Part model, mm, in its own coordinate system. Coordinates: 2 decimals unless noted, no trailing zeros. Loops run counter-clockwise (first coordinate to the right, second up) from the corner with the lowest first, then second, coordinate; pieces in that order, holes last. Notation, with made-up numbers: (52, -13.5) - (96, -13.5) arc R25 ccw to (96, 9.5) - close; hole circle Ø8 at (62, 78.25). An arc over 180 degrees is marked (long way). Use a Markdown table: item, result. Add a question column.
1. Wall check: probe 1 along Y at (x, z) = (-100, 11); probe 2 along Y at (x, z) = (100, 7.5); probe 3 along Z at (x, y) = (-183, 101). Give the ranges that are in metal, low to high. Write a range as [from, to].
2. Band-saw the part on B-B, the plane x = -150. Give the cut face in (y, z), plus the area to 3 significant figures.
3. Band-saw the part on A-A, the plane y = -60. Give the cut face in (x, z).
4. Band-saw the part on C-C, the plane x = 100. Give the cut face in (y, z).
5. Band-saw the part on D-D, the plane x = 172. Give the cut face in (y, z).
6. Pull direction Y, two halves, no side cores. Call faces 1 (the cylindrical face through (-105.5, 65.1, 12.7)), 2 (the flat face through (200, -2, 12)), 3 (the cylindrical face through (92.507, -59.67, 12.675)), 4 (the cylindrical face through (-174.977, 1.071, 27.465)): pulls with the +Y half, pulls with the -Y half, needs draft (parallel to the pull), parting line crosses it, or undercut.
7. Drop flat-ended pins along their axis: pin 1 (5 mm diameter, centred on x = -4.5, y = -51, fed in from +Z); pin 2 (2.5 mm diameter, centred on x = -131, z = 28.5, fed in from -Y); pin 3 (4.5 mm diameter, centred on y = -0.5, z = 25.5, fed in from +X). Give the stop position or say it passes through.
from build123d import *
from build123d import SkipClean  # not in build123d's __all__

# Parameters (mm, degrees)
F0_W          = 400
F0_H          = 300
F1_DEPTH      = 25
F4_R          = 25
F5_DEPTH      = 5
F6_R          = 3
F7_DEPTH      = 3
F9_END_RADIUS = 25
F8_R          = 2
F9_REACH      = 102.6578543495
F10_W         = 11.0047593287
F10_H         = 4
F11_DEPTH     = 5
F14_R         = 7.5
F15_DEPTH     = 25.001


with BuildPart() as f1:
    # F0 (on Top) → F1 (new body)
    with BuildSketch(Plane.XY):
        Rectangle(F0_W, F0_H)
    extrude(amount=F1_DEPTH)

    # F2 (on face) → F3 (revolve, cut)
    with BuildSketch(Plane.XY.offset(25)):
        Polygon((200, 0), (200, 0.5), (-100, 3), (-100, 0), align=None)
    revolve(axis=Axis((50, 0, 25), (1, 0, 0)), mode=Mode.SUBTRACT)

    # F4 (on face) → F5 (join)
    with BuildSketch(Plane.XY.offset(25)):
        with Locations((-150, 0)):
            Circle(F4_R)
    extrude(amount=F5_DEPTH)

    # F6 (on face) → F7 (cut)
    with BuildSketch(Plane.YZ.offset(-100)):
        with Locations((0, 25)):
            Circle(F6_R)
    extrude(amount=-F7_DEPTH, mode=Mode.SUBTRACT)

    f9_end = (Plane(origin=(-150, 0, 27.5), x_dir=(-1, 0, 0), z_dir=(0, 0, -1)) * Cylinder(F9_END_RADIUS, 1207.1140921674, mode=Mode.PRIVATE)).faces().sort_by_distance((-175, 0, 27.5))[0]
    # F8 (on face) → F9 (cut, up to the whole of a round face its end follows)
    with BuildSketch(Plane.YZ.offset(-103)):
        with Locations((0, 25)):
            Circle(F8_R)
    f9_long = extrude(amount=-F9_REACH, mode=Mode.PRIVATE)
    add(split(f9_long, bisect_by=f9_end, keep=Keep.ALL, mode=Mode.PRIVATE).solids().sort_by_distance((-103, 0, 25))[0], mode=Mode.SUBTRACT)

    # F10 (on face) → F11 (cut)
    with BuildSketch(Plane.XY.offset(30)):
        with Locations((-127.4976203357, 0)):
            Rectangle(F10_W, F10_H)
    extrude(amount=-F11_DEPTH, mode=Mode.SUBTRACT)

    # F12 (on face) → F13 (revolve, cut)
    with BuildSketch(Plane.XY.offset(25)):
        with BuildLine():
            Line((-133, 2), (-133, 0))
            Line((-133, 0), (-125, 0))
            ThreePointArc((-125, 0), (-125.020040135, 1.0008022485), (-125.0801284112, 2))
            Line((-125.0801284112, 2), (-133, 2))
        make_face()
        with BuildLine():
            ThreePointArc((-125.0801284112, 2), (-125.020040135, 1.0008022485), (-125, 0))
            Line((-125, 0), (-123.6437782645, 0))
            Line((-123.6437782645, 0), (-123.6437782645, 2))
            Line((-123.6437782645, 2), (-125.0801284112, 2))
        make_face()
    revolve(axis=Axis((-128.3218891323, 0, 25), (1, 0, 0)), mode=Mode.SUBTRACT)

    # F14 (on face) → F15 (cut, through all)
    with BuildSketch(Plane.XY.offset(25)):
        with Locations((100, -60)):
            Circle(F14_R)
        with Locations((-100, 60)):
            Circle(F14_R)
    extrude(amount=-F15_DEPTH, mode=Mode.SUBTRACT)


solid = f1.part
Geometry check:
| question | item | result |
|---|---|---|
| 1 | probe 1 | y = [-150, 52.5], [67.5, 150] |
| 1 | probe 2 | y = [-150, -67.5], [-52.5, 150] |
| 1 | probe 3 | z = [0, 25] |
| 2 | outline | (-150, 0) - (150, 0) - (150, 25) - (25, 25) - (25, 30) - (-25, 30) - (-25, 25) - (-150, 25) - close |
| 2 | area | 7,750 mm^2 |
| 3 | outline | (-200, 0) - (92.5, 0) - (92.5, 25) - (-200, 25) - close; (107.5, 0) - (200, 0) - (200, 25) - (107.5, 25) - close |
| 4 | outline | (-150, 0) - (-67.5, 0) - (-67.5, 25) - (-150, 25) - close; (-52.5, 0) - (150, 0) - (150, 25) - (1.33, 25) arc R1.33 cw to (-1.33, 25) - (-52.5, 25) - close |
| 5 | outline | (-150, 0) - (150, 0) - (150, 25) - (0.73, 25) arc R0.73 cw to (-0.73, 25) - (-150, 25) - close |
| 6 | face 1 | undercut |
| 6 | face 2 | needs draft |
| 6 | face 3 | undercut |
| 6 | face 4 | parting line crosses it |
| 7 | pin 1 | stops at z = 25 |
| 7 | pin 2 | stops at y = -17.61 |
| 7 | pin 3 | stops at x = 200 |
